from build123d import *

# Parameters (mm, degrees)
SKETCH_1_W                = 52
SKETCH_1_H                = 20
SKETCH_1_R                = 3
SKETCH_1_R_2              = 1.5
EXTRUDE_1_DEPTH           = 2
SKETCH_2_W                = 2
SKETCH_2_H                = 20
EXTRUDE_2_DEPTH           = 32
CUT_EXTRUDE_START         = -28
CUT_EXTRUDE_1_OUTLINE_R   = 1.5
CUT_EXTRUDE_1_OUTLINE_R_2 = 4
CUT_EXTRUDE_1_DEPTH       = 56
FILLET_1_R                = 2


# Read off the part's stored shape, not the designer's step: 切除-拉伸1
with BuildPart() as part:
    # 草图1 → 凸台-拉伸1 (new body)
    with BuildSketch(Plane(origin=(0, 0, 0), x_dir=(1, 0, 0), z_dir=(0, 1, 0))):
        Rectangle(SKETCH_1_W, SKETCH_1_H)
        with Locations(Location((0, 0, 0), (0, 0, 270))):
            Circle(SKETCH_1_R, mode=Mode.SUBTRACT)
        with Locations(Location((-4.949747468, -4.949747468, 0), (0, 0, 270))):
            Circle(SKETCH_1_R_2, mode=Mode.SUBTRACT)
        with Locations(Location((-4.949747468, 4.949747468, 0), (0, 0, 270))):
            Circle(SKETCH_1_R_2, mode=Mode.SUBTRACT)
        with Locations(Location((4.949747468, 4.949747468, 0), (0, 0, 270))):
            Circle(SKETCH_1_R_2, mode=Mode.SUBTRACT)
        with Locations(Location((4.949747468, -4.949747468, 0), (0, 0, 270))):
            Circle(SKETCH_1_R_2, mode=Mode.SUBTRACT)
        with Locations(Location((14.75, -4.949747468, 0), (0, 0, 270))):
            Circle(SKETCH_1_R_2, mode=Mode.SUBTRACT)
        with Locations(Location((14.75, 4.949747468, 0), (0, 0, 270))):
            Circle(SKETCH_1_R_2, mode=Mode.SUBTRACT)
        with Locations(Location((-14.75, -4.949747468, 0), (0, 0, 90))):
            Circle(SKETCH_1_R_2, mode=Mode.SUBTRACT)
        with Locations(Location((-14.75, 4.949747468, 0), (0, 0, 90))):
            Circle(SKETCH_1_R_2, mode=Mode.SUBTRACT)
    extrude(amount=EXTRUDE_1_DEPTH)

    # 草图2 → 凸台-拉伸2 (add)
    with BuildSketch(Plane(origin=(0, 0, 0), x_dir=(1, 0, 0), z_dir=(0, 1, 0))):
        with Locations((27, 0)):
            Rectangle(SKETCH_2_W, SKETCH_2_H)
        with Locations((-27, 0)):
            Rectangle(SKETCH_2_W, SKETCH_2_H)
    extrude(amount=EXTRUDE_2_DEPTH)

    # 切除-拉伸1 outline → 切除-拉伸1 (cut)
    with BuildSketch(Plane(origin=(0, 0, 0), x_dir=(0, 0, -1), z_dir=(1, 0, 0)).offset(CUT_EXTRUDE_START)):
        with BuildLine():
            ThreePointArc((-10, 22), (-7.071067812, 29.071067812), (0, 32))
            Line((0, 32), (-10, 32))
            Line((-10, 32), (-10, 22))
        make_face()
        with BuildLine():
            ThreePointArc((0, 32), (7.071067812, 29.071067812), (10, 22))
            Line((10, 22), (10, 32))
            Line((10, 32), (0, 32))
        make_face()
        with Locations((0, 29)):
            Circle(CUT_EXTRUDE_1_OUTLINE_R)
        with Locations((0, 15)):
            Circle(CUT_EXTRUDE_1_OUTLINE_R)
        with Locations((0, 22)):
            Circle(CUT_EXTRUDE_1_OUTLINE_R_2)
        with Locations((-7, 22)):
            Circle(CUT_EXTRUDE_1_OUTLINE_R)
        with Locations((7, 22)):
            Circle(CUT_EXTRUDE_1_OUTLINE_R)
        with Locations((-4.949747468, 17.050252532)):
            Circle(CUT_EXTRUDE_1_OUTLINE_R)
        with Locations((4.949747468, 17.050252532)):
            Circle(CUT_EXTRUDE_1_OUTLINE_R)
    extrude(amount=CUT_EXTRUDE_1_DEPTH, mode=Mode.SUBTRACT)

    # 圆角1
    fillet_1_edges = [part.edges().sort_by_distance(p)[0] for p in [
        (28, 0, 0),
        (-28, 0, 0),
    ]]
    fillet(fillet_1_edges, radius=FILLET_1_R)


solid = part.part
Geometry check sheet. Reference: the model listing, model coordinates, mm. Give positions to 0.01 mm unless a question says otherwise; leave off trailing zeros. Order: outer loops, then holes, each group sorted by start corner. A loop starts at its lowest first (then second) coordinate and runs counter-clockwise, first axis right, second up.
1. Sectioned sample at A-A (x = 14.75). Record the boundary of the cut face in (y, z), then the cut area to 3 significant figures.
Completed:
outline: (0, -10) - (2, -10) - (2, -6.45) - (0, -6.45) - close; (0, -3.45) - (2, -3.45) - (2, 3.45) - (0, 3.45) - close; (0, 6.45) - (2, 6.45) - (2, 10) - (0, 10) - close
area: 28.0 mm2
2. Depth check by flat-ended pin: pin 1 (8 mm diameter, centred on x = -3, z = 2.5, fed in from +Y). Enter the tip coordinate at first touch or a pass-through.
Completed:
pin 1: stops at y = 2
3. Scan lines: line 1 (X direction, y = 14.5, z = 2); line 2 (Y direction, x = 26.6, z = 0); line 3 (Z direction, x = -27, y = 15). Record each from-to range of solid material in increasing order.
Completed:
line 1: x = -28 to -26, 26 to 28
line 2: y = 0.09 to 13.5, 16.5 to 18, 26 to 27.5, 30.5 to 32
line 3: z = -10 to -1.5, 1.5 to 10
4. Sectioned sample at D-D (y = 15). Record the boundary of the cut face in (x, z).
Completed:
outline: (-28, -10) - (-26, -10) - (-26, -1.5) - (-28, -1.5) - close; (-28, 1.5) - (-26, 1.5) - (-26, 10) - (-28, 10) - close; (26, -10) - (28, -10) - (28, -1.5) - (26, -1.5) - close; (26, 1.5) - (28, 1.5) - (28, 10) - (26, 10) - close
5. Draft check along Z on faces 1 (the face through (26.99, 23.01, -5.89)), 2 (the face through (-27.43, 0.6, -0.14)), 3 (the face through (-27.014, 25.966, 0.521)), 4 (the face through (0, 1, 10)). Enter one of: pulls with the +Z half, pulls with the -Z half, needs draft (parallel to the pull), parting line crosses it, or undercut.
Completed:
face 1: undercut
face 2: needs draft
face 3: undercut
face 4: pulls with the +Z half
6. Sectioned sample at C-C (z = 7). Record the boundary of the cut face in (x, y), then the cut area to 3 significant figures.
Completed:
outline: (-28, 2) arc R2 ccw to (-26, 0) - (26, 0) arc R2 ccw to (28, 2) - (28, 20.5) - (26, 20.5) - (26, 2) - (-26, 2) - (-26, 20.5) - (-28, 20.5) - close; (-28, 23.5) - (-26, 23.5) - (-26, 29.14) - (-28, 29.14) - close; (26, 23.5) - (28, 23.5) - (28, 29.14) - (26, 29.14) - close
area: 207 mm2
7. Sectioned sample at B-B (y = 10.5). Record the boundary of the cut face in (x, z).
Completed:
outline: (-28, -10) - (-26, -10) - (-26, 10) - (-28, 10) - close; (26, -10) - (28, -10) - (28, 10) - (26, 10) - close
